Here's how the part is built. I have some questions about the finished solid (model axes, mm). A direction names the side the tool comes from. Coordinates: 2 decimals unless noted, no trailing zeros. Loops run counter-clockwise (first coordinate to the right, second up) from the corner with the lowest first, then second, coordinate; pieces in that order, holes last. Notation, with made-up numbers: (-18.75, -35) -> (33.25, -35) arc R32 ccw to (33.25, 4) -> close; hole circle Ø11 at (7, 49). An arc over 180 degrees is marked (long way). Answer as a JSON object with one key per item and string values. Group by question number.
1) If we mould it in two halves opening along X, with no side actions, what happens to faces 3 (the cylindrical face through (10, 3.2, 1.5)), 4 (the flat face through (0, 0, 3)), 5 (the cylindrical face through (6.86, 7, 1.48))? For each: +X half, -X half, draft (parallel to the pull), parting line (faces both ways), or undercut.
2) I need wall thicknesses on probe 1 along Y at (x, z) = (6, 0.9); probe 2 along Y at (x, z) = (1.5, 1.85); probe 3 along X at (y, z) = (8.25, 2.5). Which ranges of each line are inside material? Lowest first, please. Write a range as [from, to].
3) I want a section at C-C (x = -1). Write out the boundary of the cut face in (y, z).
4) I'm going to push flat-ended pins straight in: pin 1 (0.9 mm diameter, centred on x = -7.5, z = 1, fed in from -Y); pin 2 (1.5 mm diameter, centred on y = -7, z = 2.5, fed in from +X); pin 3 (1.5 mm diameter, centred on y = -1, z = 0.5, fed in from +X). Where does each tip first touch, or does it pass through?
5) Which directions (+Z, -Z, +X, -X, +Y, -Y) give clear straight access to the entire face, cutting with the end or side of a thin tool? Please do faces 1 (the flat face through (0, 0, 0)), 2 (the flat face through (-5, 0.4, 1)).
6) I want a section at B-B (y = 9.25). Write out the boundary of the cut face in (x, z).
7) I want a section at A-A (z = 1.35). Write out the boundary of the cut face in (x, y).
```python
from build123d import *

# Parameters (mm, degrees)
F0_R     = 10.5
F1_DEPTH = 3


with BuildPart() as f1:
    # F0 (on Top) → F1 (new body)
    with BuildSketch(Plane.XY):
        Circle(F0_R)
        with BuildLine():
            Line((-0.4, -0.4), (-0.4, -9.791833))
            ThreePointArc((-0.4, -9.791833), (-6.929646, -6.929646), (-9.791833, -0.4))
            Line((-9.791833, -0.4), (-0.4, -0.4))
        make_face(mode=Mode.SUBTRACT)
        with BuildLine():
            Line((0.4, -0.4), (9.791833, -0.4))
            ThreePointArc((9.791833, -0.4), (6.929646, -6.929646), (0.4, -9.791833))
            Line((0.4, -9.791833), (0.4, -0.4))
        make_face(mode=Mode.SUBTRACT)
        with BuildLine():
            ThreePointArc((-9.791833, 0.4), (-6.929646, 6.929646), (-0.4, 9.791833))
            Line((-0.4, 9.791833), (-0.4, 0.4))
            Line((-0.4, 0.4), (-9.791833, 0.4))
        make_face(mode=Mode.SUBTRACT)
        with BuildLine():
            Line((0.4, 0.4), (0.4, 9.791833))
            ThreePointArc((0.4, 9.791833), (6.929646, 6.929646), (9.791833, 0.4))
            Line((9.791833, 0.4), (0.4, 0.4))
        make_face(mode=Mode.SUBTRACT)
    extrude(amount=F1_DEPTH)


solid = f1.part
```
Determined:
{
 "1": {"face 3": "parting line", "face 4": "draft", "face 5": "undercut"},
 "2": {"probe 1": "[-8.62, -7.75], [-0.4, 0.4], [7.75, 8.62]", "probe 2": "[-10.39, -9.68], [-0.4, 0.4], [9.68, 10.39]", "probe 3": "[-6.5, -5.29], [-0.4, 0.4], [5.29, 6.5]"},
 "3": {"outline": "(-10.45, 0) -> (-9.75, 0) -> (-9.75, 3) -> (-10.45, 3) -> close; (-0.4, 0) -> (0.4, 0) -> (0.4, 3) -> (-0.4, 3) -> close; (9.75, 0) -> (10.45, 0) -> (10.45, 3) -> (9.75, 3) -> close"},
 "4": {"pin 1": "y = -7.78", "pin 2": "x = 8.44", "pin 3": "x = 10.5"},
 "5": {"face 1": "-Z, +X, -X, +Y, -Y", "face 2": "+Z, -Z"},
 "6": {"outline": "(-4.97, 0) -> (-3.24, 0) -> (-3.24, 3) -> (-4.97, 3) -> close; (-0.4, 0) -> (0.4, 0) -> (0.4, 3) -> (-0.4, 3) -> close; (3.24, 0) -> (4.97, 0) -> (4.97, 3) -> (3.24, 3) -> close"},
 "7": {"outline": "circle Ø21 at (0, 0); hole (-9.79, -0.4) arc R9.8 ccw to (-0.4, -9.79) -> (-0.4, -0.4) -> close; hole (-9.79, 0.4) -> (-0.4, 0.4) -> (-0.4, 9.79) arc R9.8 ccw to start; hole (0.4, -9.79) arc R9.8 ccw to (9.79, -0.4) -> (0.4, -0.4) -> close; hole (0.4, 0.4) -> (9.79, 0.4) arc R9.8 ccw to (0.4, 9.79) -> close"}
}
